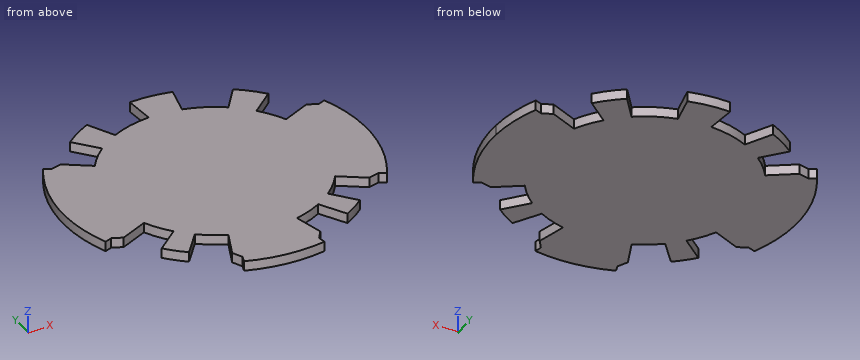
```python
from build123d import *

# Parameters (mm, degrees)
SKETCH1_R           = 35
BOSS_EXTRUDE1_DEPTH = 3.25


with BuildPart() as part:
    # Sketch1 → Boss-Extrude1 (new body)
    with BuildSketch(Plane.XY):
        Circle(SKETCH1_R)
        with BuildLine():
            Line((28.828605721, -19.847203637), (37.023656069, -25.489128697))
            ThreePointArc((37.023656069, -25.489128697), (42.922238919, -13.346467571), (44.949380312, 0))
            ThreePointArc((44.949380312, 0), (43.970183886, 9.331115657), (41.075257073, 18.255685327))
            Line((41.075257073, 18.255685327), (31.983399718, 14.214856401))
            ThreePointArc((31.983399718, 14.214856401), (34.237545109, 7.265707463), (35, 0))
            ThreePointArc((35, 0), (33.421558912, -10.392275972), (28.828605721, -19.847203637))
        make_face()
        with BuildLine():
            Line((40.598794027, -24.617047471), (42.709771039, -25.900116821))
            ThreePointArc((42.709771039, -25.900116821), (48.105442468, -13.446449287), (49.949380312, 0))
            ThreePointArc((49.949380312, 0), (49.14051871, 8.952654044), (46.74013071, 17.615356218))
            Line((46.74013071, 17.615356218), (44.429411044, 16.741820001))
            Line((44.429411044, 16.741820001), (41.075257073, 18.255685327))
            ThreePointArc((41.075257073, 18.255685327), (43.970183886, 9.331115657), (44.949380312, 0))
            ThreePointArc((44.949380312, 0), (42.922238919, -13.346467571), (37.023656069, -25.489128697))
            Line((37.023656069, -25.489128697), (40.598794027, -24.617047471))
        make_face()
        with BuildLine():
            Line((26.826271623, 22.4800167), (34.452122443, 28.870366287))
            ThreePointArc((34.452122443, 28.870366287), (30.822303091, 32.717463571), (26.765708371, 36.111544495))
            Line((26.765708371, 36.111544495), (20.716316478, 28.210534054))
            ThreePointArc((20.716316478, 28.210534054), (23.943352483, 25.528726406), (26.826271623, 22.4800167))
        make_face()
        with BuildLine():
            Line((8.489487351, 33.954802378), (10.902777017, 43.607066443))
            ThreePointArc((10.902777017, 43.607066443), (4.145424396, 44.757817719), (-2.708331204, 44.867713698))
            Line((-2.708331204, 44.867713698), (-2.108852035, 34.936409991))
            ThreePointArc((-2.108852035, 34.936409991), (3.227849925, 34.850839084), (8.489487351, 33.954802378))
        make_face()
        with BuildLine():
            ThreePointArc((-19.678070256, 40.413120907), (-24.289025087, 37.82181977), (-28.563666386, 34.70682574))
            Line((-28.563666386, 34.70682574), (-22.241203696, 27.02459728))
            ThreePointArc((-22.241203696, 27.02459728), (-18.912738555, 29.450098817), (-15.322401648, 31.467824961))
            Line((-15.322401648, 31.467824961), (-19.678070256, 40.413120907))
        make_face()
        with BuildLine():
            ThreePointArc((-37.023656069, 25.489128697), (-44.757817719, 4.145424396), (-41.075257073, -18.255685327))
            Line((-41.075257073, -18.255685327), (-31.983399718, -14.214856401))
            ThreePointArc((-31.983399718, -14.214856401), (-34.850839084, 3.227849925), (-28.828605721, 19.847203637))
            Line((-28.828605721, 19.847203637), (-37.023656069, 25.489128697))
        make_face()
        with BuildLine():
            Line((-44.429411044, -16.741820001), (-41.075257073, -18.255685327))
            ThreePointArc((-41.075257073, -18.255685327), (-44.757817719, 4.145424396), (-37.023656069, 25.489128697))
            Line((-37.023656069, 25.489128697), (-40.598794027, 24.617047471))
            Line((-40.598794027, 24.617047471), (-42.709771039, 25.900116821))
            ThreePointArc((-42.709771039, 25.900116821), (-49.736509017, 4.606545813), (-46.74013071, -17.615356218))
            Line((-46.74013071, -17.615356218), (-44.429411044, -16.741820001))
        make_face()
        with BuildLine():
            ThreePointArc((-34.452122443, -28.870366287), (-31.668184411, -31.899418279), (-28.61895911, -34.661245936))
            Line((-28.61895911, -34.661245936), (-22.284257579, -26.989106398))
            ThreePointArc((-22.284257579, -26.989106398), (-24.658548053, -24.838599154), (-26.826271623, -22.4800167))
            Line((-26.826271623, -22.4800167), (-34.452122443, -28.870366287))
        make_face()
        with BuildLine():
            ThreePointArc((-17.956374991, -41.206982267), (-4.145424396, -44.757817719), (10.082748433, -43.803937887))
            Line((10.082748433, -43.803937887), (7.850969083, -34.108097051))
            ThreePointArc((7.850969083, -34.108097051), (-3.227849925, -34.850839084), (-13.981797309, -32.085968023))
            Line((-13.981797309, -32.085968023), (-17.956374991, -41.206982267))
        make_face()
        with BuildLine():
            ThreePointArc((-17.274850221, -46.867047521), (-4.606545813, -49.736509017), (8.373275125, -49.242551286))
            Line((8.373275125, -49.242551286), (7.956694327, -46.80760748))
            Line((7.956694327, -46.80760748), (10.082748433, -43.803937887))
            ThreePointArc((10.082748433, -43.803937887), (-4.145424396, -44.757817719), (-17.956374991, -41.206982267))
            Line((-17.956374991, -41.206982267), (-16.418147872, -44.550033929))
            Line((-16.418147872, -44.550033929), (-17.274850221, -46.867047521))
        make_face()
        with BuildLine():
            Line((16.948301539, -30.622786858), (21.766161472, -39.327865505))
            ThreePointArc((21.766161472, -39.327865505), (25.270761666, -37.173046623), (28.563666386, -34.70682574))
            Line((28.563666386, -34.70682574), (22.241203696, -27.02459728))
            ThreePointArc((22.241203696, -27.02459728), (19.677171347, -28.944929224), (16.948301539, -30.622786858))
        make_face()
    extrude(amount=-BOSS_EXTRUDE1_DEPTH)


solid = part.part
```
Could you check a few things on this model? Use its own coordinates, in mm. Round coordinates to 2 decimals unless told otherwise and drop trailing zeros. Write each loop counter-clockwise with the first axis right and the second up, starting at its lowest first coordinate (ties: lowest second). Pieces come first, ordered by that corner, then holes. Notation, with made-up numbers: M 6.5,48.5 L 12.5,48.5 A32 ccw 12.5,81.5 Z; hole C -1.5,-17.5 d1. An arc over 180 degrees is marked long. Write each question's results on one line, items separated by ' | '. Start each with the question number.
1. Imagine slicing it at C-C on x = -4.5. List the corners of the cut face in (y, z) for me.
2. I need wall thicknesses on L1, parallel to Y at x = -0.5, z = -2.9; L2, parallel to X at y = 39.5, z = -1.5; L3, parallel to Y at x = -25, z = -3. Which ranges of each line are inside material? Lowest first, please. Write a range as from..to.
3. Imagine slicing it at B-B on y = 10. List the corners of the cut face in (x, z) for me.
4. Imagine slicing it at A-A on x = -24. List the corners of the cut face in (y, z) for me.
5. I'm going to push a flat-ended pin straight in: pin 1 Ø1 at (y, z) = (-34.5, -0.5) entering from -X. Where does the tip first touch, or does it pass through?
Result sheet:
1) outline: M -49.75,-3.25 L 34.71,-3.25 L 34.71,0 L -49.75,0 Z
2) L1: y = -49.95..44.95 | L2: x = -21.45..-19.23, -2.38..9.88 | L3: y = -30.28..24.49, 30.38..37.36
3) outline: M -48.94,-3.25 L 48.94,-3.25 L 48.94,0 L -48.94,0 Z
4) outline: M -29.07,-3.25 L 25.48,-3.25 L 25.48,0 L -29.07,0 Z; M 29.16,-3.25 L 38.01,-3.25 L 38.01,0 L 29.16,0 Z
5) pin 1: stops at x = -29.4
